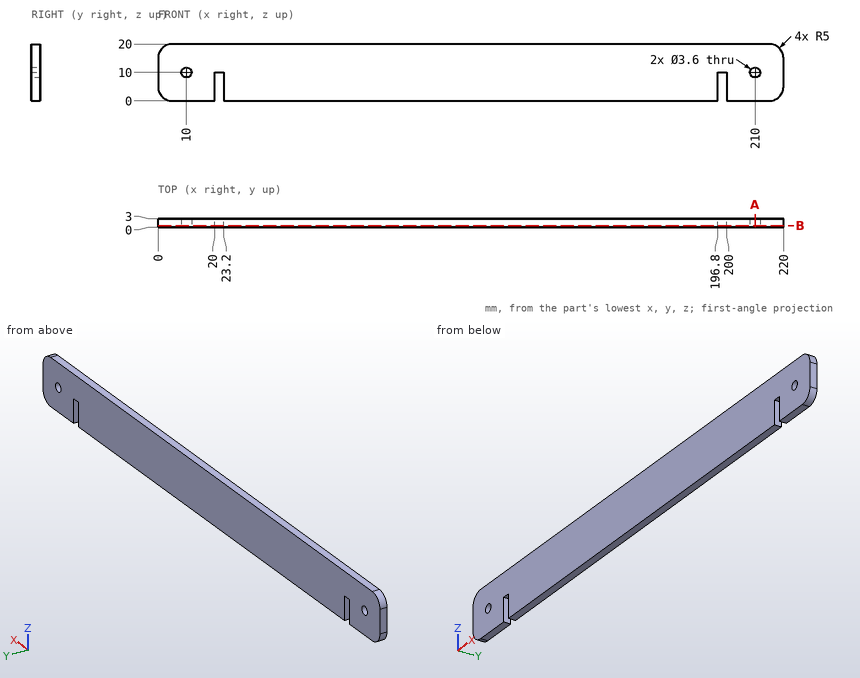
Here's the drawing with two shaded views (mm, measured from the low corner). I have some questions. Give positions to 0.01 mm unless a question says otherwise; leave off trailing zeros. Write each loop counter-clockwise with the first axis right and the second up, starting at its lowest first coordinate (ties: lowest second). Pieces come first, ordered by that corner, then holes. Notation, with made-up numbers: (20, 73) -> (61, 73) arc R21 ccw to (61, 87) -> close; hole circle Ø11 at (-28, -9). An arc over 180 degrees is marked (long way). One line per item, written item: value.
Q1. Imagine slicing it at B-B on y = 0.65. Please give me the cut outline in (x, z), and give its area (3 significant figures).
Results found:
outline: (0, 5) arc R5 ccw to (5, 0) -> (20, 0) -> (20, 10) -> (23.2, 10) -> (23.2, 0) -> (196.8, 0) -> (196.8, 10) -> (200, 10) -> (200, 0) -> (215, 0) arc R5 ccw to (220, 5) -> (220, 15) arc R5 ccw to (215, 20) -> (5, 20) arc R5 ccw to (0, 15) -> close; hole circle Ø3.6 at (10, 10); hole circle Ø3.6 at (210, 10)
area: 4,290 mm^2
Q2. Please list where these lines run through material, in increasing order: line 1 (X direction, y = 1.8, z = 5.75); line 2 (X direction, y = 2.15, z = 8.5); line 3 (Z direction, x = 210, y = 0.9). Write a range as [from, to].
Results found:
line 1: x = [0, 20], [23.2, 196.8], [200, 220]
line 2: x = [0, 9.01], [10.99, 20], [23.2, 196.8], [200, 209.01], [210.99, 220]
line 3: z = [0, 8.2], [11.8, 20]
Q3. For P1, Ø0.9, axis at y = 2, z = 2.5, coming from the -X side; P2, Ø1.5, axis at x = 198.5, y = 1, coming from the -Z side, each with a flat end and sliding along its axis, tell me the tip position at first contact or that it passes through.
Results found:
P1: stops at x = 0.44
P2: stops at z = 10
Q4. Imagine slicing it at A-A on x = 210. Please give me the cut outline in (y, z), and give its area (3 significant figures).
Results found:
outline: (0, 0) -> (3, 0) -> (3, 8.2) -> (0, 8.2) -> close; (0, 11.8) -> (3, 11.8) -> (3, 20) -> (0, 20) -> close
area: 49.2 mm^2
